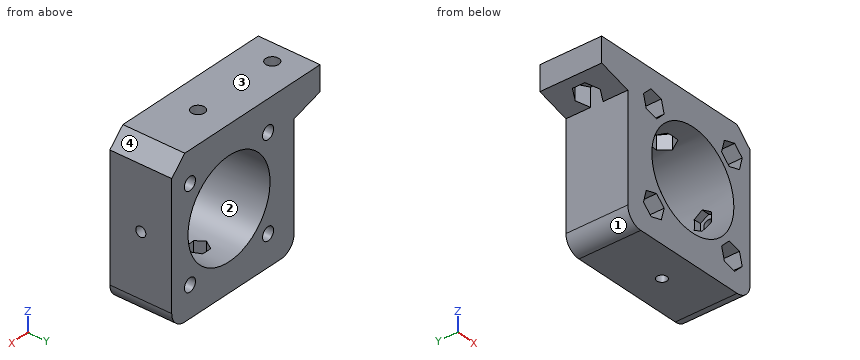
```python
from build123d import *

# Parameters (mm, degrees)
CROQUIS1_R               = 2.125
CROQUIS1_R_2             = 15.75
SALIENTE_EXTRUIR1_DEPTH  = 20
CORTAR_EXTRUIR1_REACH    = 66.226
CROQUIS3_R               = 2.125
CORTAR_EXTRUIR2_REACH    = 71.226
CORTAR_EXTRUIR2_START    = -5
CORTAR_EXTRUIR3_DEPTH    = 10
SKETCH1_W                = 3
SKETCH1_H                = 60
CUT_EXTRUDE1_DEPTH       = 48.434164903
REDONDEO1_R              = 5
CUT_EXTRUDE2_DEPTH       = 48.434164903
SKETCH3_R                = 1.625
CUT_EXTRUDE3_DEPTH       = 10
CUT_EXTRUDE4_REACH       = 71.376
CUT_EXTRUDE4_END_RADIUS  = 15.75
CUT_EXTRUDE4_START       = -4
CUT_EXTRUDE5_REACH       = 66.226
CUT_EXTRUDE5_END_RADIUS  = 15.75
SKETCH5_R                = 1.625
CUT_EXTRUDE6_REACH       = 70.226
CUT_EXTRUDE6_END_RADIUS  = 15.75
CUT_EXTRUDE6_START       = -4
REDONDEO1_OF_SIMETR_A1_R = 5
CROQUIS6_W               = 57
CROQUIS6_H               = 20
CORTAR_EXTRUIR4_DEPTH    = 73.972597597
CROQUIS7_W               = 57
CROQUIS7_H               = 20
CORTAR_EXTRUIR5_DEPTH    = 73.972597597


with BuildPart() as part:
    # Croquis1 → Saliente-Extruir1 (new body)
    with BuildSketch(Plane(origin=(0, 0, 0), x_dir=(1, 0, 0), z_dir=(0, 1, 0))):
        Polygon((25, 25), (-25, 25), (-25, -14), (-35, -17), (-35, -25), (25, -25), align=None)
        with Locations(Location((-15, -15, 0), (0, 0, 270))):
            Circle(CROQUIS1_R, mode=Mode.SUBTRACT)
        with Locations(Location((15, -15, 0), (0, 0, 270))):
            Circle(CROQUIS1_R, mode=Mode.SUBTRACT)
        with Locations(Location((-15, 15, 0), (0, 0, 270))):
            Circle(CROQUIS1_R, mode=Mode.SUBTRACT)
        with Locations(Location((0, 0, 0), (0, 0, 270))):
            Circle(CROQUIS1_R_2, mode=Mode.SUBTRACT)
        with Locations(Location((15, 15, 0), (0, 0, 270))):
            Circle(CROQUIS1_R, mode=Mode.SUBTRACT)
    saliente_extruir1 = extrude(amount=-SALIENTE_EXTRUIR1_DEPTH)

    # Croquis3 → Cortar-Extruir1 (cut, up to next)
    with BuildSketch(Plane.XY.offset(25), mode=Mode.PRIVATE) as cortar_extruir1_sk1:
        with Locations((-28.5, -10)):
            Circle(CROQUIS3_R)
    cortar_extruir1_tool1 = extrude(cortar_extruir1_sk1.sketch, amount=-CORTAR_EXTRUIR1_REACH, mode=Mode.PRIVATE) & part.part
    # Croquis3 → Cortar-Extruir1 (cut, up to next)
    with BuildSketch(Plane.XY.offset(25), mode=Mode.PRIVATE) as cortar_extruir1_sk2:
        with Locations((0, -10)):
            Circle(CROQUIS3_R)
    cortar_extruir1_tool2 = extrude(cortar_extruir1_sk2.sketch, amount=-CORTAR_EXTRUIR1_REACH, mode=Mode.PRIVATE) & part.part
    cortar_extruir1_1 = cortar_extruir1_tool1.solids().sort_by_distance((-28.5, -10, 25))[0]
    add(cortar_extruir1_1, mode=Mode.SUBTRACT)
    cortar_extruir1_2 = cortar_extruir1_tool2.solids().sort_by_distance((0, -10, 25))[0]
    add(cortar_extruir1_2, mode=Mode.SUBTRACT)
    cortar_extruir1 = cortar_extruir1_1 + cortar_extruir1_2  # Cortar-Extruir1 as one shape, for the pattern or mirror that repeats it

    # Croquis4 → Cortar-Extruir2 (cut, up to next)
    with BuildSketch(Plane.XY.offset(25).offset(CORTAR_EXTRUIR2_START), mode=Mode.PRIVATE) as cortar_extruir2_sk1:
        Polygon((-28.5, -14.041451884), (-25, -12.020725942), (-25, -7.979274058), (-28.5, -5.958548116), (-32, -7.979274058), (-32, -12.020725942), align=None)
    cortar_extruir2_tool1 = extrude(cortar_extruir2_sk1.sketch, amount=-CORTAR_EXTRUIR2_REACH, mode=Mode.PRIVATE) & part.part
    # Croquis4 → Cortar-Extruir2 (cut, up to next)
    with BuildSketch(Plane.XY.offset(25).offset(CORTAR_EXTRUIR2_START), mode=Mode.PRIVATE) as cortar_extruir2_sk2:
        Polygon((2.020725942, -13.5), (4.041451884, -10), (2.020725942, -6.5), (-2.020725942, -6.5), (-4.041451884, -10), (-2.020725942, -13.5), align=None)
    cortar_extruir2_tool2 = extrude(cortar_extruir2_sk2.sketch, amount=-CORTAR_EXTRUIR2_REACH, mode=Mode.PRIVATE) & part.part
    cortar_extruir2_1 = cortar_extruir2_tool1.solids().sort_by_distance((-28.5, -10, 20))[0]
    add(cortar_extruir2_1, mode=Mode.SUBTRACT)
    cortar_extruir2_2 = cortar_extruir2_tool2.solids().sort_by_distance((0, -10, 20))[0]
    add(cortar_extruir2_2, mode=Mode.SUBTRACT)
    cortar_extruir2 = cortar_extruir2_1 + cortar_extruir2_2  # Cortar-Extruir2 as one shape, for the pattern or mirror that repeats it

    # Croquis5 → Cortar-Extruir3 (cut)
    with BuildSketch(Plane.XZ.offset(20)):
        Polygon((-11.040489496, 13.939052358), (-12.101437138, 17.898562862), (-16.060947642, 18.959510504), (-18.959510504, 16.060947642), (-17.898562862, 12.101437138), (-13.939052358, 11.040489496), align=None)
        Polygon((11.040489496, 13.939052358), (13.939052358, 11.040489496), (17.898562862, 12.101437138), (18.959510504, 16.060947642), (16.060947642, 18.959510504), (12.101437138, 17.898562862), align=None)
        Polygon((-13.939052358, -11.040489496), (-17.898562862, -12.101437138), (-18.959510504, -16.060947642), (-16.060947642, -18.959510504), (-12.101437138, -17.898562862), (-11.040489496, -13.939052358), align=None)
        Polygon((18.959510504, -16.060947642), (17.898562862, -12.101437138), (13.939052358, -11.040489496), (11.040489496, -13.939052358), (12.101437138, -17.898562862), (16.060947642, -18.959510504), align=None)
    cortar_extruir3 = extrude(amount=-CORTAR_EXTRUIR3_DEPTH, mode=Mode.SUBTRACT)

    # Sketch1 → Cut-Extrude1 (cut, through all)
    with BuildSketch(Plane(origin=(0, 0, 0), x_dir=(1, 0, 0), z_dir=(0, 1, 0))):
        with Locations((23.5, 5)):
            Rectangle(SKETCH1_W, SKETCH1_H)
    cut_extrude1 = extrude(amount=-CUT_EXTRUDE1_DEPTH, mode=Mode.SUBTRACT)

    # Redondeo1
    redondeo1_edges = [part.edges().sort_by_distance(p)[0] for p in [
        (22, -10, -25),
        (-25, -10, -25),
    ]]
    fillet(redondeo1_edges, radius=REDONDEO1_R)

    # Sketch2 → Cut-Extrude2 (cut, through all)
    with BuildSketch(Plane(origin=(0, 0, 0), x_dir=(1, 0, 0), z_dir=(0, 1, 0))):
        Polygon((22, -25), (22, -20), (17, -25), align=None)
    cut_extrude2 = extrude(amount=-CUT_EXTRUDE2_DEPTH, mode=Mode.SUBTRACT)

    # Sketch3 → Cut-Extrude3 (cut)
    with BuildSketch(Plane(origin=(22, 0, 0), x_dir=(0, 0, -1), z_dir=(1, 0, 0))):
        with Locations((0, -10)):
            Circle(SKETCH3_R)
    cut_extrude3 = extrude(amount=-CUT_EXTRUDE3_DEPTH, mode=Mode.SUBTRACT)

    # Cut-Extrude4: up to this cylinder (the profile starts outside it)
    cut_extrude4_end = Plane(origin=(0, -10, 0), z_dir=(0, 1, 0)) * Cylinder(CUT_EXTRUDE4_END_RADIUS, 175.252, mode=Mode.PRIVATE)
    # Sketch4 → Cut-Extrude4 (cut, up to the surface)
    with BuildSketch(Plane(origin=(22, 0, 0), x_dir=(0, 0, -1), z_dir=(1, 0, 0)).offset(CUT_EXTRUDE4_START), mode=Mode.PRIVATE) as cut_extrude4_sk1:
        Polygon((1.58771324, -12.75), (3.175426481, -10), (1.58771324, -7.25), (-1.58771324, -7.25), (-3.175426481, -10), (-1.58771324, -12.75), align=None)
    cut_extrude4_tool1 = extrude(cut_extrude4_sk1.sketch, amount=-CUT_EXTRUDE4_REACH, mode=Mode.PRIVATE) - cut_extrude4_end
    cut_extrude4 = cut_extrude4_tool1.solids().sort_by_distance((18, -10, 0))[0]
    add(cut_extrude4, mode=Mode.SUBTRACT)

    # Cut-Extrude5: up to this cylinder (the profile starts outside it)
    cut_extrude5_end = Plane(origin=(0, -10, 0), z_dir=(0, 1, 0)) * Cylinder(CUT_EXTRUDE5_END_RADIUS, 164.952, mode=Mode.PRIVATE)
    # Sketch5 → Cut-Extrude5 (cut, up to the surface)
    with BuildSketch(Plane(origin=(0, 0, -25), x_dir=(-1, 0, 0), z_dir=(0, 0, -1)), mode=Mode.PRIVATE) as cut_extrude5_sk1:
        with Locations((0, -10)):
            Circle(SKETCH5_R)
    cut_extrude5_tool1 = extrude(cut_extrude5_sk1.sketch, amount=-CUT_EXTRUDE5_REACH, mode=Mode.PRIVATE) - cut_extrude5_end
    cut_extrude5 = cut_extrude5_tool1.solids().sort_by_distance((0, -10, -25))[0]
    add(cut_extrude5, mode=Mode.SUBTRACT)

    # Cut-Extrude6: up to this cylinder (the profile starts outside it)
    cut_extrude6_end = Plane(origin=(0, -10, 0), z_dir=(0, 1, 0)) * Cylinder(CUT_EXTRUDE6_END_RADIUS, 172.952, mode=Mode.PRIVATE)
    # Sketch6 → Cut-Extrude6 (cut, up to the surface)
    with BuildSketch(Plane(origin=(0, 0, -25), x_dir=(-1, 0, 0), z_dir=(0, 0, -1)).offset(CUT_EXTRUDE6_START), mode=Mode.PRIVATE) as cut_extrude6_sk1:
        Polygon((1.58771324, -12.75), (3.175426481, -10), (1.58771324, -7.25), (-1.58771324, -7.25), (-3.175426481, -10), (-1.58771324, -12.75), align=None)
    cut_extrude6_tool1 = extrude(cut_extrude6_sk1.sketch, amount=-CUT_EXTRUDE6_REACH, mode=Mode.PRIVATE) - cut_extrude6_end
    cut_extrude6 = cut_extrude6_tool1.solids().sort_by_distance((0, -10, -21))[0]
    add(cut_extrude6, mode=Mode.SUBTRACT)

    # Simetría1: Saliente-Extruir1, Cortar-Extruir1, Cortar-Extruir2, Cortar-Extruir3, Cut-Extrude1, Cut-Extrude2, Cut-Extrude3, Cut-Extrude4, Cut-Extrude5, Cut-Extrude6 across plane
    add(saliente_extruir1.mirror(Plane.ZX.offset(-20)))
    add(cortar_extruir1.mirror(Plane.ZX.offset(-20)), mode=Mode.SUBTRACT)
    add(cortar_extruir2.mirror(Plane.ZX.offset(-20)), mode=Mode.SUBTRACT)
    add(cortar_extruir3.mirror(Plane.ZX.offset(-20)), mode=Mode.SUBTRACT)
    add(cut_extrude1.mirror(Plane.ZX.offset(-20)), mode=Mode.SUBTRACT)
    add(cut_extrude2.mirror(Plane.ZX.offset(-20)), mode=Mode.SUBTRACT)
    add(cut_extrude3.mirror(Plane.ZX.offset(-20)), mode=Mode.SUBTRACT)
    add(cut_extrude4.mirror(Plane.ZX.offset(-20)), mode=Mode.SUBTRACT)
    add(cut_extrude5.mirror(Plane.ZX.offset(-20)), mode=Mode.SUBTRACT)
    add(cut_extrude6.mirror(Plane.ZX.offset(-20)), mode=Mode.SUBTRACT)

    # Redondeo1 of Simetría1
    redondeo1_of_simetr_a1_edges = [part.edges().sort_by_distance(p)[0] for p in [
        (22, -30, -25),
        (-25, -30, -25),
    ]]
    fillet(redondeo1_of_simetr_a1_edges, radius=REDONDEO1_OF_SIMETR_A1_R)

    # Croquis6 → Cortar-Extruir4 (cut, through all)
    with BuildSketch(Plane(origin=(0, 0, -25), x_dir=(-1, 0, 0), z_dir=(0, 0, -1))):
        with Locations((6.5, -10)):
            Rectangle(CROQUIS6_W, CROQUIS6_H)
    extrude(amount=-CORTAR_EXTRUIR4_DEPTH, mode=Mode.SUBTRACT)

    # Simetría4: part across plane


with BuildPart() as part_1:
    add(part.part)
    add(part.part.mirror(Plane(origin=(22, -20, 25), x_dir=(0, 0, 1), z_dir=(0, -1, 0))))

    # Croquis7 → Cortar-Extruir5 (cut, through all)
    with BuildSketch(Plane(origin=(0, 0, -25), x_dir=(-1, 0, 0), z_dir=(0, 0, -1))):
        with Locations((6.5, -30)):
            Rectangle(CROQUIS7_W, CROQUIS7_H)
    extrude(amount=-CORTAR_EXTRUIR5_DEPTH, mode=Mode.SUBTRACT)


solid = part_1.part
```
For this review, take the finished solid that the model builds, in its own axes (mm). Face numbers are marked on the shaded views. Round coordinates to 2 decimals unless told otherwise and drop trailing zeros. Write each loop counter-clockwise with the first axis right and the second up, starting at its lowest first coordinate (ties: lowest second). Pieces come first, ordered by that corner, then holes. Notation, with made-up numbers: (-5, 37) - (7, 37) arc R6 cw to (7, 43) - close; hole circle Ø11 at (-21, 65). An arc over 180 degrees is marked (long way). Put each result on its own line as item: value.
Q1. Mouldability with a two-part tool opening along X and no side actions: class the marked faces 1, 2, 3 and 4 as released by +X, released by -X, zero draft, split by the parting line, or undercut.
Solved:
face 1: released by -X
face 2: undercut
face 3: zero draft
face 4: released by +X
Q2. We need section C-C (x = -15). Give the boundary of the cut face in (y, z) (3 decimals), and give its area (3 significant figures).
Solved:
outline: (-20, -25) - (0, -25) - (0, -17.125) - (-10, -17.125) - (-10, -18.675) - (-20, -18.675) - close; (-20, -11.325) - (-10, -11.325) - (-10, -12.875) - (0, -12.875) - (0, -4.802) - (-20, -4.802) - close; (-20, 4.802) - (0, 4.802) - (0, 12.875) - (-10, 12.875) - (-10, 11.325) - (-20, 11.325) - close; (-20, 18.675) - (-10, 18.675) - (-10, 17.125) - (0, 17.125) - (0, 25) - (-20, 25) - close
area: 576 mm2
Q3. Insertion check: pin 1 Ø2 at (y, z) = (-16, -10.5) entering from -X; pin 2 Ø4 at (x, y) = (-23.5, -3.5) entering from -Z; pin 3 Ø2.5 at (x, z) = (15, 13.5) entering from -Y; pin 4 Ø2 at (x, z) = (-3, -12.5) entering from +Y. Each pin has a flat end and moves straight along its axis. Give the tip position at first contact, or say it passes through.
Solved:
pin 1: stops at x = -25
pin 2: stops at z = -24.77
pin 3: stops at y = -10
pin 4: passes through
Q4. We need section B-B (z = 0). Give the boundary of the cut face in (x, y) (3 decimals), and give its area (3 significant figures).
Solved:
outline: (-25, -20) - (-15.75, -20) - (-15.75, 0) - (-25, 0) - close; (15.75, -20) - (22, -20) - (22, -11.625) - (18, -11.625) - (18, -12.75) - (15.75, -12.75) - close; (15.75, -7.25) - (18, -7.25) - (18, -8.375) - (22, -8.375) - (22, 0) - (15.75, 0) - close
area: 285 mm2
Q5. We need section D-D (z = 8). Give the boundary of the cut face in (x, y), and give its area (3 significant figures).
Solved:
outline: (-25, -20) - (-13.57, -20) - (-13.57, 0) - (-25, 0) - close; (13.57, -20) - (22, -20) - (22, 0) - (13.57, 0) - close
area: 397 mm2
Q6. Wall thickness on probe 1 along Y at (x, z) = (0, -17.5); probe 2 along Z at (x, y) = (-13, -15.75); probe 3 along Y at (x, z) = (0, 23.35) (3 decimals): over which ranges is each line inside the solid? List them lowest first.
Solved:
probe 1: y = -20 to -12.75, -7.25 to 0
probe 2: z = -25 to -18.14, -11.98 to -8.89, 8.89 to 11.98, 18.14 to 25
probe 3: y = -20 to -12.125, -7.875 to 0
Q7. We need section A-A (y = -15.25). Count the separate pieces of the cut face and the enclosed holes in it, and give its area (3 significant figures).
Solved:
separate pieces: 1
enclosed holes: 5
area: 1,470 mm2
